Can you work these out from the drawing? Everything is in mm from the part's minimum corner. A direction names the side the tool comes from. Round coordinates to 2 decimals unless told otherwise and drop trailing zeros. Order: outer loops, then holes, each group sorted by start corner. A loop starts at its lowest first (then second) coordinate and runs counter-clockwise, first axis right, second up. Notation, with made-up numbers: (-3.5, -18) - (15.5, -18) arc R17 ccw to (15.5, 4) - close; hole circle Ø9 at (85, -13.5). An arc over 180 degrees is marked (long way). Answer as a JSON object with one key per item and string values.
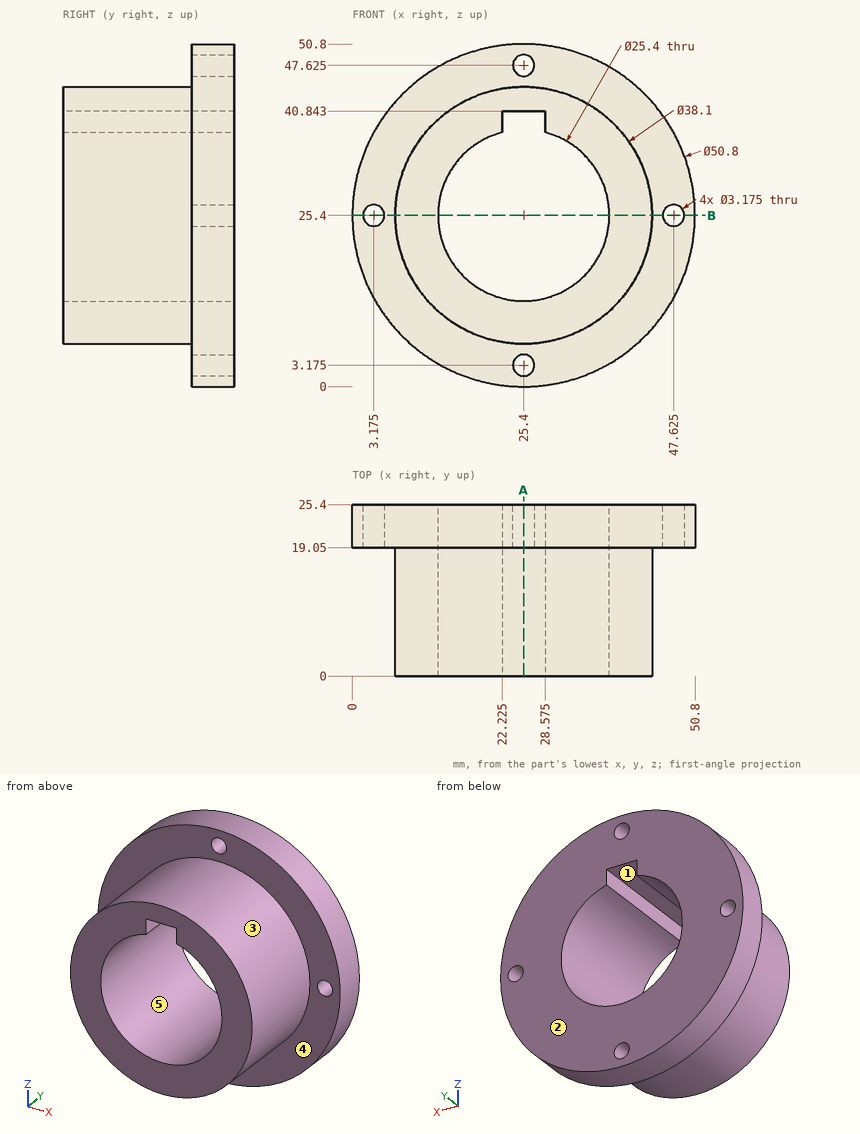
1. For P1, Ø1.6, axis at y = 16, z = 40, coming from the +X side; P2, Ø4, axis at x = 25.4, z = 47.625, coming from the +Y side; P3, Ø3, axis at y = 15, z = 11, coming from the -X side; P4, Ø6, axis at x = 43.5, z = 12.5, coming from the -Y side, each with a flat end and sliding along its axis, tell me the tip position at first contact or that it passes through.
Responses:
{"P1": "x = 38.53", "P2": "y = 25.4", "P3": "x = 11.38", "P4": "y = 19.05"}
2. Thinking about a two-plate mould opening in Z: for the marked faces 3, 4 and 5, which applies, pulls with the +Z half, pulls with the -Z half, needs draft (parallel to the pull), parting line crosses it, or undercut?
Responses:
{"face 3": "parting line crosses it", "face 4": "needs draft", "face 5": "undercut"}
3. For the marked faces 1 and 2, which set-ups out of +Z, -Z, +X, -X, +Y, -Y let a thin tool reach every point of the face, with its end or its side?
Responses:
{"face 1": "+Y, -Y", "face 2": "+Z, -Z, +X, -X, +Y"}
4. If I drill on L1, parallel to Z at x = 25.4, y = 22; L2, parallel to X at y = 23.5, z = 25; L3, parallel to Y at x = 45, z = 26, over which ranges is the centre line in solid material (lowest first)? Write a range as [from, to].
Responses:
{"L1": "[0, 1.59], [4.76, 12.7], [40.84, 46.04], [49.21, 50.8]", "L2": "[0, 1.64], [4.71, 12.71], [38.09, 46.09], [49.16, 50.8]", "L3": "[19.05, 25.4]"}
5. Imagine slicing it at A-A (x = 25.4). List the corners of the cut face in (y, z) for me.
Responses:
{"outline": "(0, 6.35) - (19.05, 6.35) - (19.05, 4.76) - (25.4, 4.76) - (25.4, 12.7) - (0, 12.7) - close; (0, 40.84) - (25.4, 40.84) - (25.4, 46.04) - (19.05, 46.04) - (19.05, 44.45) - (0, 44.45) - close; (19.05, 0) - (25.4, 0) - (25.4, 1.59) - (19.05, 1.59) - close; (19.05, 49.21) - (25.4, 49.21) - (25.4, 50.8) - (19.05, 50.8) - close"}
6. Imagine slicing it at B-B (z = 25.4). List the corners of the cut face in (x, y) for me, plus the area to 3 significant figures.
Responses:
{"outline": "(0, 19.05) - (1.59, 19.05) - (1.59, 25.4) - (0, 25.4) - close; (4.76, 19.05) - (6.35, 19.05) - (6.35, 0) - (12.7, 0) - (12.7, 25.4) - (4.76, 25.4) - close; (38.1, 0) - (44.45, 0) - (44.45, 19.05) - (46.04, 19.05) - (46.04, 25.4) - (38.1, 25.4) - close; (49.21, 19.05) - (50.8, 19.05) - (50.8, 25.4) - (49.21, 25.4) - close", "area": "363 mm2"}
